Job drawing, mm, ordinate dimensions from the low corner. One solid piece. A direction names the side the tool comes from. Round coordinates to 2 decimals unless told otherwise and drop trailing zeros. Loops run counter-clockwise (first coordinate to the right, second up) from the corner with the lowest first, then second, coordinate; pieces in that order, holes last.
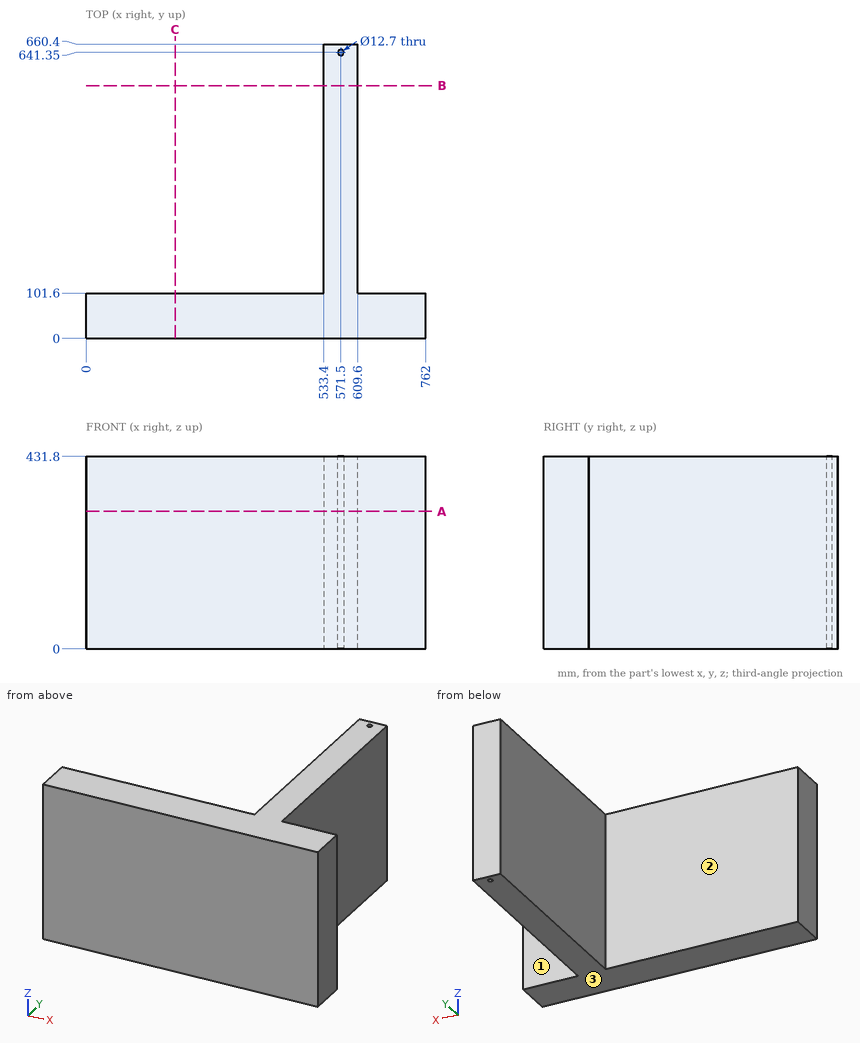
1) Slice it at B-B, the plane y = 567. Give the cut face in (x, z), then the cut area to 3 significant figures.
Values:
outline: (533.4, 0) - (609.6, 0) - (609.6, 431.8) - (533.4, 431.8) - close
area: 32,900 mm2
2) Drop flat-ended pins along their axis: pin 1 Ø5 at (x, y) = (643, 82) entering from -Z; pin 2 Ø3 at (y, z) = (375, 376) entering from -X; pin 3 Ø6 at (x, z) = (429.5, 52.5) entering from +Y; pin 4 Ø3 at (y, z) = (132.5, 212.5) entering from +X. Give the stop position or say it passes through.
Values:
pin 1: stops at z = 0
pin 2: stops at x = 533.4
pin 3: stops at y = 101.6
pin 4: stops at x = 609.6
3) Wall check: line 1 along Y through (x, z) = (571.5, 118.5); line 2 along X through (y, z) = (641, 103); line 3 along Y through (x, z) = (108, 366). Give the ranges that are in metal, low to high.
Values:
line 1: y = 0 to 635, 647.7 to 660.4
line 2: x = 533.4 to 565.16, 577.84 to 609.6
line 3: y = 0 to 101.6
4) Slice it at A-A, the plane z = 308.5. Give the cut face in (x, y).
Values:
outline: (0, 0) - (762, 0) - (762, 101.6) - (609.6, 101.6) - (609.6, 660.4) - (533.4, 660.4) - (533.4, 101.6) - (0, 101.6) - close; hole circle Ø12.7 at (571.5, 641.35)
5) Tool access for the marked faces 1, 2 and 3: list every direction of +Z, -Z, +X, -X, +Y, -Y with a clear straight run to the whole face (end or side of a thin tool).
Values:
face 1: +Z, -Z, +X, +Y
face 2: +Z, -Z, -X, +Y
face 3: -Z, +X, -X, +Y, -Y
6) Slice it at C-C, the plane x = 200. Give the cut face in (y, z), then the cut area to 3 significant figures.
Values:
outline: (0, 0) - (101.6, 0) - (101.6, 431.8) - (0, 431.8) - close
area: 43,900 mm2
